```python
from build123d import *

# Parameters (mm, degrees)
BOSS_EXTRU_1_DEPTH              = 4
DIAM_TRE_DU_PER_AGE_6_1_6_1_1_D = 6.1
CONG_1_R                        = 1


with BuildPart() as part:
    # Esquisse1 → Boss.-Extru.1 (new body)
    with BuildSketch(Plane(origin=(0, 2, 0), x_dir=(1, 0, 0), z_dir=(0, 0, -1))):
        with BuildLine():
            Line((-31, -1), (31, -1))
            ThreePointArc((31, -1), (40, 2), (31, 5))
            Line((31, 5), (-31, 5))
            ThreePointArc((-31, 5), (-40, 2), (-31, -1))
        make_face()
    extrude(amount=-BOSS_EXTRU_1_DEPTH)

    # Diamètre du perçage Ø6.1 (6.1)1 (through all)
    with Locations(Plane(origin=(0, 0, 4), x_dir=(-1, 0, 0), z_dir=(0, 0, 1))):
        with Locations((35, 0)):
            Hole(DIAM_TRE_DU_PER_AGE_6_1_6_1_1_D / 2)

    # Esquisse4 → Fraisage pour vis à tête fraisée M2.51 (revolve, cut)
    with BuildSketch(Plane(origin=(35, 0, 4), x_dir=(0, -1, 0), z_dir=(1, 0, 0))):
        Polygon((0, 0), (0, 4), (3.3, 4), (1.5, 2.2), (1.5, 1.8), (3.3, 0), align=None)
    revolve(axis=Axis((35, 0, 10.35), (0, 0, -1)), mode=Mode.SUBTRACT)

    # Congé1
    cong_1_edges = [part.edges().sort_by_distance(p)[0] for p in [
        (40, 0, 4),
        (0, -3, 4),
        (-40, 0, 4),
        (0, -3, 0),
        (40, 0, 0),
        (0, 3, 0),
        (-40, 0, 0),
        (0, 3, 4),
    ]]
    fillet(cong_1_edges, radius=CONG_1_R)


solid = part.part
```
Geometry: final body of the model. Coordinates: model frame, mm. A direction names the side the tool comes from. Round coordinates to 2 decimals unless told otherwise and drop trailing zeros. Write each loop counter-clockwise with the first axis right and the second up, starting at its lowest first coordinate (ties: lowest second). Pieces come first, ordered by that corner, then holes. Notation, with made-up numbers: M 67,20.25 L 92,20.25 A27 ccw 92,51.25 Z; hole C -39.75,-5.75 d9. An arc over 180 degrees is marked long. Answer in a Markdown table with one row per item. Add a question column.
(1) Draft query along X for faces 4 (the face through (36.464, 0.325, 2.003)), 5 (the face through (-1, 0, 4)). Return one class per face: pulls with the +X half, pulls with the -X half, needs draft (parallel to the pull), parting line crosses it, or undercut.
(2) Contact query for flat-ended pins moving along their axis: pin 1 (1 mm diameter, centred on x = 0, z = 1.5, fed in from +Y); pin 2 (2 mm diameter, centred on x = 1, z = 1.5, fed in from -Y). Output: stop coordinate, or through.
(3) Cut plane C-C, the plane x = 35. Return the cut outline in (y, z).
(4) Reachability of faces 1 (the face through (0, 3, 2)), 2 (the face through (0, -3, 2)), 3 (the face through (-40, 0, 2)) from +Z, -Z, +X, -X, +Y, -Y: full face, straight path, thin tool, end or side. Return the list, or none.
(5) Cut plane B-B, the plane x = -35. Return the cut outline in (y, z).
(6) Ray query, L1, parallel to Y at x = -35, z = 1.4; L2, parallel to X at y = -0.25, z = 1.3; L3, parallel to X at y = 1.5, z = 1.65. Return the intervals inside material, ascending.
(7) Cut plane A-A, the plane y = 0. Return the cut outline in (x, z), then the cut area to 3 significant figures.
(8) Cut plane D-D, the plane x = -22. Return the cut outline in (y, z).
Established:
| question | item | result |
|---|---|---|
| 1 | face 4 | undercut |
| 1 | face 5 | needs draft |
| 2 | pin 1 | y = 3 |
| 2 | pin 2 | y = -3 |
| 3 | outline | M -5,1 A1 ccw -4,0 L -3.3,0 L -1.5,1.8 L -1.5,2.2 L -3.3,4 L -4,4 A1 ccw -5,3 Z; M 1.5,1.8 L 3.3,0 L 4,0 A1 ccw 5,1 L 5,3 A1 ccw 4,4 L 3.3,4 L 1.5,2.2 Z |
| 4 | face 1 | +Z, -Z, +Y |
| 4 | face 2 | +Z, -Z, -Y |
| 4 | face 3 | +Z, -Z |
| 5 | outline | M -5,1 A1 ccw -4,0 L -3.05,0 L -3.05,4 L -4,4 A1 ccw -5,3 Z; M 3.05,0 L 4,0 A1 ccw 5,1 L 5,3 A1 ccw 4,4 L 3.05,4 Z |
| 6 | L1 | -5 to -3.05, 3.05 to 5 |
| 6 | L2 | -39.99 to -38.04, -31.96 to 33.02, 36.98 to 39.99 |
| 6 | L3 | -39.77 to -37.66, -32.34 to 34.31, 35.69 to 39.77 |
| 7 | outline | M -40,1 A1 ccw -39,0 L -38.05,0 L -38.05,4 L -39,4 A1 ccw -40,3 Z; M -31.95,0 L 31.7,0 L 33.5,1.8 L 33.5,2.2 L 31.7,4 L -31.95,4 Z; M 36.5,1.8 L 38.3,0 L 39,0 A1 ccw 40,1 L 40,3 A1 ccw 39,4 L 38.3,4 L 36.5,2.2 Z |
| 7 | area | 276 mm² |
| 8 | outline | M -3,1 A1 ccw -2,0 L 2,0 A1 ccw 3,1 L 3,3 A1 ccw 2,4 L -2,4 A1 ccw -3,3 Z |
